Autodesk Inventor part; units mm, degrees
ref_plane "Work Plane1" through (-5.1816, 0, -12.2936) normal (1, 0, 0) x (0, 0, -1)
ref_plane "Work Plane2" through (-14.7066, 0, -12.2936) normal (1, 0, 0) x (0, 0, -1)
ref_plane "YZ Plane" through (0, 0, 0) normal (1, 0, 0) x (0, 1, 0)
sketch "Sketch1" plane through (0, 0, 0) normal (0, 1, 0) x (-1, 0, 0)
  line L0 (0, 0) -> (30.0482, 0)
  line L1 (30.0482, 0) -> (30.0482, -24.13)
  line L2 (30.0482, -24.13) -> (0, -24.13)
  line L3 (0, -24.13) -> (0, 0)
  line L4 (5.1816, -12.2936) -> (5.1816, -20.8026) construction
  line L5 (3.7719, -12.2936) -> (3.7719, -20.8026)
  line L6 (6.5913, -20.8026) -> (6.5913, -12.2936)
  arc A0 (6.5913, -12.2936) -> (3.7719, -12.2936) centre (5.1816, -12.2936) ccw
  arc A1 (3.7719, -20.8026) -> (6.5913, -20.8026) centre (5.1816, -20.8026) ccw
  line L7 (14.7066, -12.2936) -> (14.7066, -20.8026) construction
  line L8 (13.2969, -12.2936) -> (13.2969, -20.8026)
  line L9 (16.1163, -20.8026) -> (16.1163, -12.2936)
  arc A2 (16.1163, -12.2936) -> (13.2969, -12.2936) centre (14.7066, -12.2936) ccw
  arc A3 (13.2969, -20.8026) -> (16.1163, -20.8026) centre (14.7066, -20.8026) ccw
  line L10 (26.4414, -4.4958) -> (3.6068, -4.4958) construction
  line L11 (26.4414, -2.7958) -> (3.6068, -2.7958)
  line L12 (3.6068, -6.1958) -> (26.4414, -6.1958)
  arc A4 (26.4414, -6.1958) -> (26.4414, -2.7958) centre (26.4414, -4.4958) ccw
  arc A5 (3.6068, -2.7958) -> (3.6068, -6.1958) centre (3.6068, -4.4958) ccw
  point P0 (5.1816, -16.5481)
  point P1 (14.7066, -16.5481)
  point P2 (15.0241, -4.4958)
  dimension "d0" = 30.0482
  dimension "d1" = 24.13
  dimension "d5" = 12.2936
  dimension "d6" = 2.8194
  dimension "d7" = 5.1816
  dimension "d8" = 3.3274
  dimension "d11" = 9.525
  dimension "d16" = 3.4
  dimension "d17" = 4.4958
  dimension "d18" = 3.6068
  dimension "d19" = 3.6068
extrude "Extrusion1" add sketch "Sketch1" along normal blind 2.54
sketch "Sketch2" plane through (0, 2.54, 0) normal (0, 1, 0) x (1, 0, 0)
  line L0 (0, 24.13) -> (-30.0482, 24.13)
  line L1 (0, 0) -> (0, 24.13)
  line L2 (-30.0482, 24.13) -> (0, 24.13)
  line L3 (0, 24.13) -> (0, 9.5)
  line L4 (0, 9.5) -> (-30.0482, 9.5)
  line L5 (-30.0482, 9.5) -> (-30.0482, 24.13)
  line L6 (-30.0482, 0) -> (0, 0)
  line L7 (-1.8161, 9.5) -> (-1.8161, 24.13)
  line L8 (-1.8161, 24.13) -> (-8.5471, 24.13)
  line L9 (-8.5471, 24.13) -> (-8.5471, 9.5)
  arc A0 (-6.5913, 12.2936) -> (-3.7719, 12.2936) centre (-5.1816, 12.2936) ccw
  line L10 (-8.5471, 0.4572) -> (-1.8161, 24.13) construction
  line L11 (-1.8161, 0.4572) -> (-8.5471, 24.13) construction
  line L12 (-8.5471, 9.5) -> (-1.5875, 9.5)
  line L13 (-18.0721, 24.13) -> (-18.0721, 9.5)
  line L14 (-11.3411, 9.5) -> (-11.3411, 24.13)
  line L15 (-18.0721, 9.5) -> (-11.1125, 9.5)
  line L16 (-11.3411, 24.13) -> (-18.0721, 24.13)
  point P0 (-8.5471, 9.5)
  point P1 (-18.0721, 9.5)
  dimension "d22" = 9.5
  dimension "d23" = 6.731
  dimension "d24" = 3.3655
  dimension "d27" = 9.525
extrude "Extrusion2" add sketch "Sketch2" along normal blind 3.937 contours L1 L4 L7 L0 | L9 L4 L14 L0 | L13 L4 L5 L0
ref_plane "Work Plane1" through (-5.1816, 0, -12.2936) normal (1, 0, 0) x (0, 0, -1)
ref_plane "Work Plane2" through (-14.7066, 0, -12.2936) normal (1, 0, 0) x (0, 0, -1)
sketch "Sketch3" plane through (0, 0, 0) normal (1, 0, 0) x (0, 0, -1)
  line L0 (24.13, 6.477) -> (9.5, 6.477)
  line L1 (24.13, 6.477) -> (21.59, 6.477)
  line L2 (21.59, 6.477) -> (21.59, 5.207)
  line L3 (21.59, 5.207) -> (24.13, 5.207)
  line L4 (24.13, 5.207) -> (24.13, 6.477)
  point P0 (0, 0)
  dimension "d35" = 2.54
  dimension "d36" = 1.27
extrude "Extrusion3" cut sketch "Sketch3" against normal through all
fillet "Fillet2" radius 3.175 4 edges at (0, 1.27, 0) (0, 2.6035, -24.13) (-30.0482, 2.6035, -24.13) (-30.0482, 1.27, 0)
equation "\"d19\" = d18"
equation "\"d27\" = d11"
properties part number "Limit switch mount top nut well"
For this review, take the finished solid that the model builds, in its own axes (mm). A direction names the side the tool comes from. Round coordinates to 2 decimals unless told otherwise and drop trailing zeros. Order: outer loops, then holes, each group sorted by start corner. A loop starts at its lowest first (then second) coordinate and runs counter-clockwise, first axis right, second up. Notation, with made-up numbers: (85.5, -9.75) -> (93.5, -9.75) arc R25 ccw to (93.5, 7.25) -> close; hole circle Ø4 at (37, 38.25). An arc over 180 degrees is marked (long way). Put each result on its own line as item: value.
Q1. Machinability: for faces 1 (the flat face through (-11.341, 4, -17)), 2 (the flat face through (-13.297, 1, -16)), 3 (the flat face through (-24, 4, -9.5)), 4 (the flat face through (-24, 5.207, -23)), which of the approach directions +Z, -Z, +X, -X, +Y, -Y give a long, thin tool a straight path to every point of the face, cutting with its end or side? Answer none if there is none.
Check result:
face 1: +Z, -Z, +Y
face 2: +Y, -Y
face 3: +Z, +X, -X, +Y
face 4: -Z, +X, -X, +Y
Q2. For probe 1 along X at (y, z) = (3.5, -20.75); probe 2 along Z at (x, y) = (-11, 1.75); probe 3 along Z at (x, y) = (-13.5, 0.75), list the stretches that pass through material, from the lowest coordinate up. Write a range as [from, to].
Check result:
probe 1: [-30.05, -18.07], [-11.34, -8.55], [-1.82, 0]
probe 2: [-24.13, -6.2], [-2.8, 0]
probe 3: [-24.13, -21.53], [-11.56, -6.2], [-2.8, 0]
Q3. Insertion check: pin 1 Ø1.5 at (y, z) = (4.5, -16.5) entering from +X; pin 2 Ø1.4 at (x, y) = (-10.5, 6) entering from -Z; pin 3 Ø1.9 at (x, z) = (-1.5, -23) entering from +Y; pin 4 Ø1.5 at (x, y) = (-3.5, 5) entering from -Z. Each pin has a flat end and moves straight along its axis. Give the tip position at first contact, or say it passes through.
Check result:
pin 1: x = 0
pin 2: z = -21.59
pin 3: y = 5.21
pin 4: through
Q4. Add section D-D on y = 1.25. Write out the cut boundary in (x, z) (3 decimals).
Check result:
outline: (-30.048, -20.955) arc R3.175 ccw to (-26.873, -24.13) -> (-3.175, -24.13) arc R3.175 ccw to (0, -20.955) -> (0, -3.175) arc R3.175 ccw to (-3.175, 0) -> (-26.873, 0) arc R3.175 ccw to (-30.048, -3.175) -> close; hole (-26.441, -6.196) -> (-3.607, -6.196) arc R1.7 ccw to (-3.607, -2.796) -> (-26.441, -2.796) arc R1.7 ccw to start; hole (-16.116, -20.803) arc R1.41 ccw to (-13.297, -20.803) -> (-13.297, -12.294) arc R1.41 ccw to (-16.116, -12.294) -> close; hole (-6.591, -20.803) arc R1.41 ccw to (-3.772, -20.803) -> (-3.772, -12.294) arc R1.41 ccw to (-6.591, -12.294) -> close
Q5. Add section B-B on y = 3.5. State how many separate pieces and enclosed holes the cut face has, plus the area to 3 significant figures.
Check result:
separate pieces: 3
enclosed holes: 0
area: 238 mm2
Q6. Add section A-A on x = -25. Write out the cut boundary in (y, z), plus the area to 3 significant figures.
Check result:
outline: (0, -24.13) -> (5.21, -24.13) -> (5.21, -21.59) -> (6.48, -21.59) -> (6.48, -9.5) -> (2.54, -9.5) -> (2.54, -6.2) -> (0, -6.2) -> close; (0, -2.8) -> (2.54, -2.8) -> (2.54, 0) -> (0, 0) -> close
area: 107 mm2
Q7. Add section C-C on z = -19.75. Write out the cut boundary in (x, y), plus the area to 3 significant figures.
Check result:
outline: (-30.05, 0) -> (-16.12, 0) -> (-16.12, 2.54) -> (-18.07, 2.54) -> (-18.07, 6.48) -> (-30.05, 6.48) -> close; (-13.3, 0) -> (-6.59, 0) -> (-6.59, 2.54) -> (-8.55, 2.54) -> (-8.55, 6.48) -> (-11.34, 6.48) -> (-11.34, 2.54) -> (-13.3, 2.54) -> close; (-3.77, 0) -> (0, 0) -> (0, 6.48) -> (-1.82, 6.48) -> (-1.82, 2.54) -> (-3.77, 2.54) -> close
area: 127 mm2
